from build123d import *

# Parameters (mm, degrees)
F0_W     = 65.873436
F0_H     = 34.102622
F1_DEPTH = 51.9


with BuildPart() as f1:
    # F0 (on Top) → F1 (new body)
    with BuildSketch(Plane.XY):
        Polygon((-32.936718, 17.051311), (32.936718, 17.051311), (0, 49.113605), align=None)
        Rectangle(F0_W, F0_H)
    extrude(amount=F1_DEPTH)


solid = f1.part
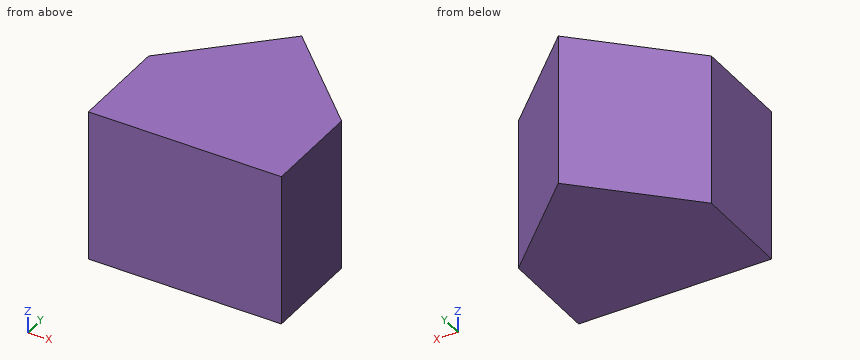
Geometry check sheet. Reference: the model listing, model coordinates, mm. Round coordinates to 2 decimals unless told otherwise and drop trailing zeros. Loops run counter-clockwise (first coordinate to the right, second up) from the corner with the lowest first, then second, coordinate; pieces in that order, holes last.
Item 1: Thickness scan on line 1 (Y direction, x = 11, z = 27.5); line 2 (Y direction, x = 29, z = 20); line 3 (X direction, y = 45, z = 16). Record the ranges inside material, lowest first.
Item 2: Cross-section at C-C on y = 28.5. Record the boundary of the cut face in (x, z).
Item 3: Gauge pin test, flat ends, axial feed: pin 1 (12 mm diameter, centred on x = 15, z = 6, fed in from +Y); pin 2 (6 mm diameter, centred on x = -24, z = 46, fed in from +Y); pin 3 (12 mm diameter, centred on x = -6, y = -1, fed in from -Z); pin 4 (6 mm diameter, centred on y = 35, z = 28.5, fed in from -X). Record the tip position at first contact, or that the pin passes through.
Item 4: Cross-section at B-B on x = -12.5. Record the boundary of the cut face in (y, z), then the cut area to 3 significant figures.
Item 5: Cross-section at A-A on z = 42. Record the boundary of the cut face in (x, y).
Answer sheet:
1. line 1: y = -17.05 to 38.41
1. line 2: y = -17.05 to 20.88
1. line 3: x = -4.23 to 4.23
2. outline: (-21.18, 0) - (21.18, 0) - (21.18, 51.9) - (-21.18, 51.9) - close
3. pin 1: stops at y = 40.35
3. pin 2: stops at y = 28.67
3. pin 3: stops at z = 0
3. pin 4: stops at x = -17.58
4. outline: (-17.05, 0) - (36.95, 0) - (36.95, 51.9) - (-17.05, 51.9) - close
4. area: 2,800 mm2
5. outline: (-32.94, -17.05) - (32.94, -17.05) - (32.94, 17.05) - (0, 49.11) - (-32.94, 17.05) - close
